from build123d import *

# Parameters (mm, degrees)
F0_R     = 11.75
F0_R_2   = 1.7
F1_DEPTH = 76.36
F2_R     = 2
F3_START = -2
F3_DEPTH = 2.35
F4_DEPTH = 89.7
F6_START = -2
F5_R     = 1.7
F6_DEPTH = 2.5


with BuildPart() as f1:
    # F0 (on Front) → F1 (new body)
    with BuildSketch(Plane.XZ):
        Circle(F0_R)
        Polygon((1.6112496617, 2.7362762765), (3.175309598, -0.0272450006), (1.5640599363, -2.7635212771), (-1.6112496617, -2.7362762765), (-3.175309598, 0.0272450006), (-1.5640599363, 2.7635212771), align=None, mode=Mode.SUBTRACT)
        Polygon((1.5640599363, -2.7635212771), (3.175309598, -0.0272450006), (1.6112496617, 2.7362762765), (-1.5640599363, 2.7635212771), (-3.175309598, 0.0272450006), (-1.6112496617, -2.7362762765), align=None)
        Circle(F0_R_2, mode=Mode.SUBTRACT)
        Circle(F0_R_2)
    extrude(amount=-F1_DEPTH)

    # F2
    f2_edges = [f1.edges().sort_by_distance(p)[0] for p in [
        (-11.75, 0, 0),
        (-11.75, 76.36, 0),
    ]]
    fillet(f2_edges, radius=F2_R)

    # F0 (on Front) → F3 (cut)
    with BuildSketch(Plane.XZ.offset(F3_START)):
        Polygon((1.5640599363, -2.7635212771), (3.175309598, -0.0272450006), (1.6112496617, 2.7362762765), (-1.5640599363, 2.7635212771), (-3.175309598, 0.0272450006), (-1.6112496617, -2.7362762765), align=None)
        Circle(F0_R_2, mode=Mode.SUBTRACT)
    extrude(amount=-F3_DEPTH, mode=Mode.SUBTRACT)

    # F0 (on Front) → F4 (cut)
    with BuildSketch(Plane.XZ):
        Circle(F0_R_2)
    extrude(amount=-F4_DEPTH, mode=Mode.SUBTRACT)

    # F5 (on face) → F6 (cut)
    with BuildSketch(Plane(origin=(0, 76.36, 0), x_dir=(-1, 0, 0), z_dir=(0, 1, 0)).offset(F6_START)):
        Polygon((-1.5877132403, -2.75), (1.5877132403, -2.75), (3.1754264805, 0), (1.5877132403, 2.75), (-1.5877132403, 2.75), (-3.1754264805, 0), align=None)
        Circle(F5_R, mode=Mode.SUBTRACT)
    extrude(amount=-F6_DEPTH, mode=Mode.SUBTRACT)


solid = f1.part
Geometry check sheet. Reference: the model listing, model coordinates, mm. A direction names the side the tool comes from. Coordinates: 2 decimals unless noted, no trailing zeros. Order: outer loops, then holes, each group sorted by start corner. A loop starts at its lowest first (then second) coordinate and runs counter-clockwise, first axis right, second up. Notation, with made-up numbers: (22.25, 61.5) - (66.25, 61.5) arc R18 ccw to (66.25, 70.5) - close; hole circle Ø8 at (-9, 19.5). An arc over 180 degrees is marked (long way). Answer in a Markdown table with one row per item. Add a question column.
1) Cross-section at A-A, the plane y = 45.5. Record the cut outline in (x, z).
2) Gauge pin test, flat ends, axial feed: P1, Ø4, axis at y = 29.5, z = 4, coming from the -X side; P2, Ø1, axis at y = 29.5, z = -2.5, coming from the +X side; P3, Ø3, axis at x = 0, z = 0, coming from the -Y side; P4, Ø1.5, axis at x = 3, y = 22.5, coming from the -Z side. Record the tip position at first contact, or that the pin passes through.
3) Set-up check for faces 4 (the cylindrical face through (-0.37, 37.63, -1.66)), 5 (the flat face through (2.4, 3.16, 1.34)): record each of +Z, -Z, +X, -X, +Y, -Y from which the full face is reachable in a straight line by a thin tool's end or side.
4) Release check for a two-part mould opening along X. For faces 1 (the flat face through (1.4, 2, 1.3)), 2 (the flat face through (0, 0, -2)), 3 (the cylindrical face through (11.207, 37.673, 3.529)) record: +X half, -X half, draft (parallel to the pull), parting line (faces both ways), or undercut.
5) Material ranges on line 1 along Y through (x, z) = (0.5, -2.25); line 2 along Z through (x, y) = (0, 75.3); line 3 along Z through (x, y) = (0, 36.5), recorded low to high. Write a range as [from, to].
6) Cross-section at B-B, the plane x = 0. Record the cut outline in (y, z), then the cut area to 3 significant figures.
Check result:
| question | item | result |
|---|---|---|
| 1 | outline | circle Ø23.5 at (0, 0); hole circle Ø3.4 at (0, 0) |
| 2 | P1 | stops at x = -11.58 |
| 2 | P2 | stops at x = 11.58 |
| 2 | P3 | passes through |
| 2 | P4 | stops at z = -11.53 |
| 3 | face 4 | +Y, -Y |
| 3 | face 5 | none |
| 4 | face 1 | undercut |
| 4 | face 2 | draft |
| 4 | face 3 | parting line |
| 5 | line 1 | y = [0, 2], [4.35, 71.86], [74.36, 76.36] |
| 5 | line 2 | z = [-11.52, -1.7], [1.7, 11.52] |
| 5 | line 3 | z = [-11.75, -1.7], [1.7, 11.75] |
| 6 | outline | (0, -9.75) arc R2 ccw to (2, -11.75) - (74.36, -11.75) arc R2 ccw to (76.36, -9.75) - (76.36, -1.7) - (74.36, -1.7) - (74.36, -2.75) - (71.86, -2.75) - (71.86, -1.7) - (4.35, -1.7) - (4.35, -2.75) - (2, -2.75) - (2, -1.7) - (0, -1.7) - close; (0, 1.7) - (2, 1.7) - (2, 2.75) - (4.35, 2.75) - (4.35, 1.7) - (71.86, 1.7) - (71.86, 2.75) - (74.36, 2.75) - (74.36, 1.7) - (76.36, 1.7) - (76.36, 9.75) arc R2 ccw to (74.36, 11.75) - (2, 11.75) arc R2 ccw to (0, 9.75) - close |
| 6 | area | 1,520 mm² |
